Source: CAD feature listing. Evaluate the final solid. Frame: model axes, mm. Face numbers are marked on the shaded views. Round coordinates to 2 decimals unless told otherwise and drop trailing zeros. Write each loop counter-clockwise with the first axis right and the second up, starting at its lowest first coordinate (ties: lowest second). Pieces come first, ordered by that corner, then holes. Notation, with made-up numbers: M -27,50.5 L 2,50.5 A26 cw 2,84.5 Z; hole C -22.5,79.25 d2. An arc over 180 degrees is marked long. Use a Markdown table: item, result.
```python
from build123d import *

# Parameters (mm, degrees)
F0_W     = 40
F0_H     = 50
F1_DEPTH = 2
F2_W     = 40
F2_H     = 50
F2_W_2   = 36
F2_H_2   = 46
F3_DEPTH = 3
F4_W     = 38.5
F4_H     = 48.5
F4_W_2   = 36
F4_H_2   = 46
F5_DEPTH = 1.3
F6_W     = 32
F6_H     = 0.75
F7_DEPTH = 1.3


with BuildPart() as f1:
    # F0 (on Front) → F1 (new body)
    with BuildSketch(Plane.XZ):
        Rectangle(F0_W, F0_H)
    extrude(amount=F1_DEPTH)

    # F2 (on face) → F3 (join)
    with BuildSketch(Plane.XZ.offset(2)):
        Rectangle(F2_W, F2_H)
        Rectangle(F2_W_2, F2_H_2, mode=Mode.SUBTRACT)
    extrude(amount=F3_DEPTH)

    # F4 (on face) → F5 (cut)
    with BuildSketch(Plane.XZ.offset(5)):
        Rectangle(F4_W, F4_H)
        Rectangle(F4_W_2, F4_H_2, mode=Mode.SUBTRACT)
    extrude(amount=-F5_DEPTH, mode=Mode.SUBTRACT)

    # F6 (on face) → F7 (cut)
    with BuildSketch(Plane.XZ.offset(5)):
        with Locations((0, -24.625)):
            Rectangle(F6_W, F6_H)
    extrude(amount=-F7_DEPTH, mode=Mode.SUBTRACT)


solid = f1.part
```
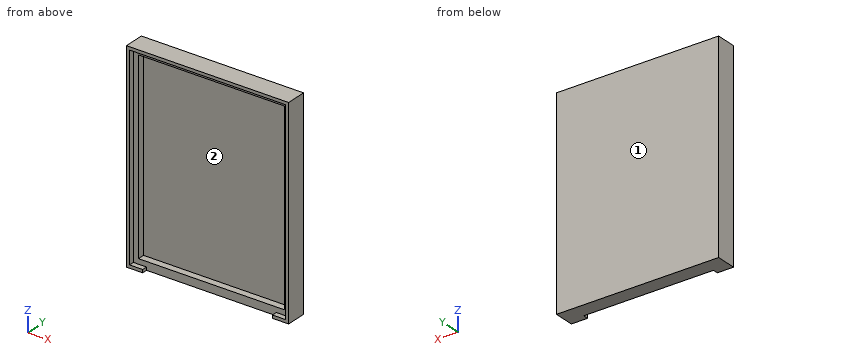
Q1. Section B-B on z = 7. Return loops of the section in (x, y), plus the area to 4 significant figures.
Results are:
| item | result |
|---|---|
| outline | M -20,-5 L -19.25,-5 L -19.25,-3.7 L -18,-3.7 L -18,-2 L 18,-2 L 18,-3.7 L 19.25,-3.7 L 19.25,-5 L 20,-5 L 20,0 L -20,0 Z |
| area | 88.75 mm^2 |
Q2. First-contact query: pin 1 Ø11.5 at (x, z) = (-4, -10.5) entering from -Y; pin 2 Ø0.6 at (x, y) = (-6, -4.5) entering from -Z. Flat tips, straight axial feed; report the tip coordinate or a pass-through.
Results are:
| item | result |
|---|---|
| pin 1 | y = -2 |
| pin 2 | z = 24.25 |
Q3. Line query: L1, parallel to Z at x = -4, y = -3.6; L2, parallel to X at y = -3, z = 0.5; L3, parallel to X at y = -4.55, z = 0. Output: solid intervals per line, ascending.
Results are:
| item | result |
|---|---|
| L1 | -25 to -23, 23 to 25 |
| L2 | -20 to -18, 18 to 20 |
| L3 | -20 to -19.25, 19.25 to 20 |
Q4. Section A-A on x = 9. Return loops of the section in (y, z).
Results are:
| item | result |
|---|---|
| outline | M -5,24.25 L -3.7,24.25 L -3.7,23 L -2,23 L -2,-23 L -3.7,-23 L -3.7,-25 L 0,-25 L 0,25 L -5,25 Z |
Q5. Mould query, pull axis X, two halves, no side actions, for the marked faces 1 and 2. Classes: +X half, -X half, draft (parallel to the pull), parting line (faces both ways), or undercut.
Results are:
| item | result |
|---|---|
| face 1 | draft |
| face 2 | undercut |
Q6. Section C-C on y = -2.95. Return loops of the section in (x, z), plus the area to 3 significant figures.
Results are:
| item | result |
|---|---|
| outline | M -20,-25 L 20,-25 L 20,25 L -20,25 Z; hole M -18,-23 L 18,-23 L 18,23 L -18,23 Z |
| area | 344 mm^2 |
